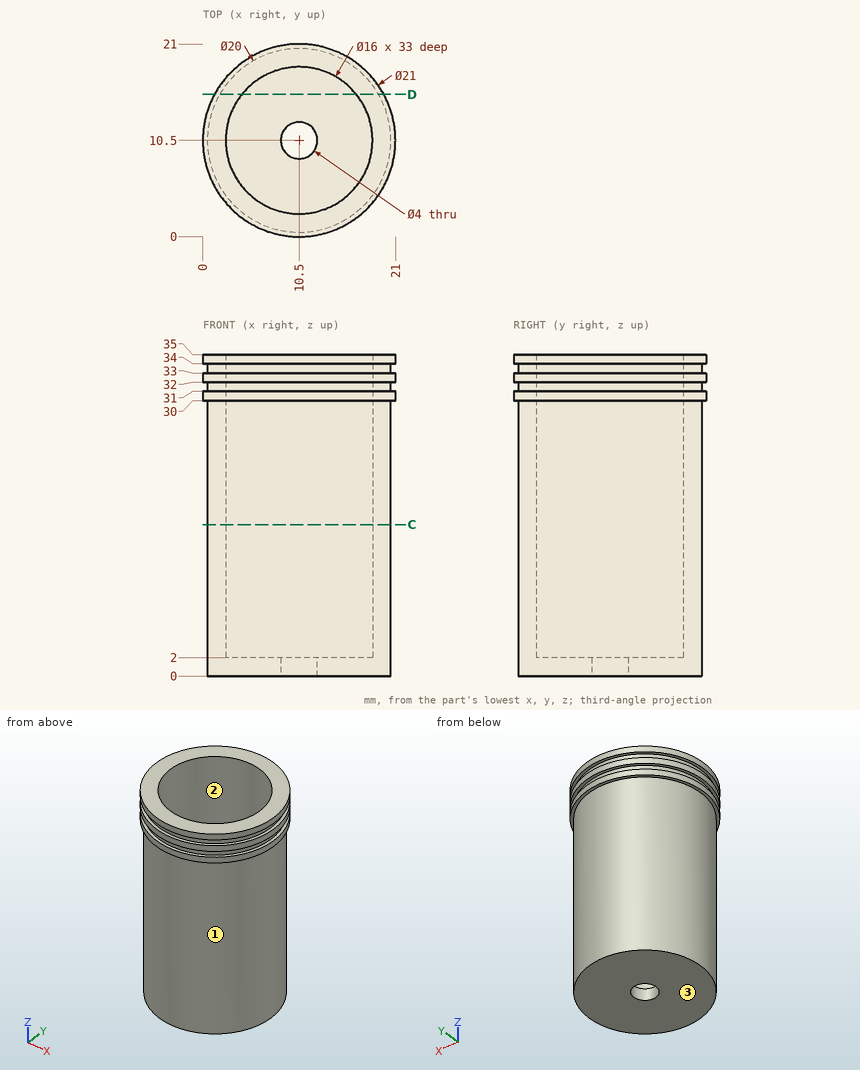
Source: three-view drawing plus pictorial views. Frame: mm from the lowest corner of the part. Round coordinates to 2 decimals unless told otherwise and drop trailing zeros. Loops run counter-clockwise (first coordinate to the right, second up) from the corner with the lowest first, then second, coordinate; pieces in that order, holes last.
Q1. Section C-C, the plane z = 16.5. Return loops of the section in (x, y).
Q2. Mould query, pull axis X, two halves, no side actions, for the marked faces 1, 2 and 3. Classes: pulls with the +X half, pulls with the -X half, needs draft (parallel to the pull), parting line crosses it, or undercut.
Q3. Section D-D, the plane y = 15.5. Return loops of the section in (x, z) (3 decimals).
Q4. First-contact query: P1, Ø4, axis at y = 14.5, z = 31.5, coming from the +X side; P2, Ø1, axis at x = 13, y = 17.5, coming from the +Z side; P3, Ø6, axis at x = 13, z = 15.5, coming from the +Y side. Flat tips, straight axial feed; report the tip coordinate or a pass-through.
Q5. Ray query, line 1 (Z direction, x = 19.5, y = 15.25); line 2 (Y direction, x = 10.5, z = 28); line 3 (Y direction, x = 10.5, z = 1.25). Return the intervals inside material, ascending.
Solutions:
1. outline: circle Ø20 at (10.5, 10.5); hole circle Ø16 at (10.5, 10.5)
2. face 1: parting line crosses it
2. face 2: undercut
2. face 3: needs draft
3. outline: (1.267, 30) - (1.84, 30) - (1.84, 0) - (19.16, 0) - (19.16, 30) - (19.733, 30) - (19.733, 31) - (19.16, 31) - (19.16, 32) - (19.733, 32) - (19.733, 33) - (19.16, 33) - (19.16, 34) - (19.733, 34) - (19.733, 35) - (16.745, 35) - (16.745, 2) - (4.255, 2) - (4.255, 35) - (1.267, 35) - (1.267, 34) - (1.84, 34) - (1.84, 33) - (1.267, 33) - (1.267, 32) - (1.84, 32) - (1.84, 31) - (1.267, 31) - close
4. P1: stops at x = 20.8
4. P2: stops at z = 2
4. P3: stops at y = 20.5
5. line 1: z = 30 to 31, 32 to 33, 34 to 35
5. line 2: y = 0.5 to 2.5, 18.5 to 20.5
5. line 3: y = 0.5 to 8.5, 12.5 to 20.5
